Solid Edge part; units mm, degrees
sketch "Sketch1" plane through (0, 0, 0) normal (0, -1, 0) x (1, 0, 0)
  line L0 (-13.5, 0) -> (13.5, 0)
  line L1 (13.5, 0) -> (13.5, 90)
  line L2 (13.5, 90) -> (-13.5, 90)
  line L3 (-13.5, 90) -> (-13.5, 0)
  dimension "D1" = 13.5
  dimension "D2" = 13.5
extrude "Protrusion1" add sketch "Sketch1" against normal blind 17
sketch "Sketch2" plane through (0, 17, 40) normal (0, 1, 0) x (-1, 0, 0)
  line L0 (-10.5, -30) -> (10.5, -30)
  line L1 (10.5, -30) -> (10.5, 11)
  line L2 (10.5, 11) -> (-10.5, 11)
  line L3 (-10.5, 11) -> (-10.5, -30)
  dimension "D1" = 10.5
  dimension "D2" = 10.5
extrude "ExtrudedCutout_1" cut sketch "Sketch2" against normal blind 53.489
sketch "Sketch3" plane through (0, 17, 40) normal (0, 1, 0) x (-1, 0, 0)
  line L0 (-4.432, 40.7205) -> (-1.9698, 26.7205)
  arc A0 (-1.9698, 26.7205) -> (1.9698, 26.7205) centre (0, 27.067) ccw
  line L1 (4.432, 40.7205) -> (1.9698, 26.7205)
  arc A1 (-4.432, 40.7205) -> (4.432, 40.7205) centre (0, 41.5) cw
  dimension "D1" = 4.432
extrude "ExtrudedCutout_2" cut sketch "Sketch3" against normal blind 5
fillet "Round_1" radius 6 4 edges at (-13.5, 8.5, 0) (13.5, 8.5, 0) (13.5, 8.5, 90) (-13.5, 8.5, 90)
sketch "Sketch4" plane through (0, 12, 75.5335) normal (0, 1, 0) x (-0.1732, 0, -0.9849)
  circle A0 centre (-5.8763, 1.0335) radius 1
extrude "Cutout1" cut sketch "Sketch4" against normal through all
sketch "Sketch5" plane through (0, 0, 45) normal (0, -1, 0) x (0, 0, 1)
  circle A0 centre (36.5, 0) radius 4.5
extrude "ExtrudedCutout_4" cut sketch "Sketch5" against normal blind 8.5833
sketch "Sketch6" plane through (0, 0, 45) normal (0, -1, 0) x (0, 0, -1)
  line L0 (17.05, 13.5) -> (32.05, 13.5)
  line L1 (32.05, 13.5) -> (32.05, 10.5)
  line L2 (32.05, 10.5) -> (17.05, 10.5)
  line L3 (17.05, 10.5) -> (17.05, 13.5)
  line L4 (17.05, -10.5) -> (32.05, -10.5)
  line L5 (32.05, -10.5) -> (32.05, -13.5)
  line L6 (32.05, -13.5) -> (17.05, -13.5)
  line L7 (17.05, -13.5) -> (17.05, -10.5)
  dimension "D1" = 17.05
extrude "ExtrudedProtrusion_3" add sketch "Sketch6" along normal blind 12
sketch "Sketch7" plane through (-12, -12, 20.45) normal (0, -1, 0) x (0, 0, -1)
  line L0 (-7.5, -1.5) -> (7.5, -1.5)
  line L1 (7.5, -1.5) -> (7.5, 25.5)
  line L2 (7.5, 25.5) -> (-7.5, 25.5)
  line L3 (-7.5, 25.5) -> (-7.5, -1.5)
extrude "ExtrudedProtrusion_4" add sketch "Sketch7" along normal blind 3.4534
sketch "Sketch8" plane through (0, -15.4534, 20.45) normal (0, -1, 0) x (1, 0, 0)
  circle A0 centre (0, 0) radius 1.5
extrude "ExtrudedCutout_5" cut sketch "Sketch8" against normal blind 4.5945
fillet "Round_2" radius 6 3 edges at (-12, 0, 27.95) (12, 0, 27.95) (-12, 0, 12.95)
Input: part model. Units: mm. Frame: model coordinates. A direction names the side the tool comes from. Coordinates: 2 decimals unless noted, no trailing zeros. Loops run counter-clockwise (first coordinate to the right, second up) from the corner with the lowest first, then second, coordinate; pieces in that order, holes last. Notation, with made-up numbers: (75.25, -7) - (99.25, -7) arc R31 cw to (99.25, 28) - close; hole circle Ø10 at (66.5, 89). An arc over 180 degrees is marked (long way). Answer in a Markdown table with one row per item. Add a question column.
Item 1: Contact query for flat-ended pins moving along their axis: P1, Ø7.5, axis at x = -3, z = 22.5, coming from the +Y side; P2, Ø2.5, axis at x = 0, z = 81.5, coming from the -Y side; P3, Ø10, axis at x = 0, z = 82.5, coming from the -Y side. Output: stop coordinate, or through.
Item 2: Section query B-B on y = 3.5. Return the cut outline in (x, z).
Item 3: Section query C-C on x = 3.25. Return the cut outline in (y, z).
Item 4: Mould query, pull axis Z, two halves, no side actions, for faces 5 (the flat face through (0, -13, 27.95)), 6 (the flat face through (0, 8.583, 83)), 7 (the cylindrical face through (-11.696, 8.619, 1.711)). Classes: released by +Z, released by -Z, zero draft, split by the parting line, or undercut.
Item 5: Access query for faces 1 (the flat face through (0, 9, 51)), 2 (the flat face through (0, 0, 4)), 3 (the flat face through (-3.22, 14.54, 73.82)), 4 (the cylindrical face through (-11.789, 8.619, 88.196)). Directions: +Z, -Z, +X, -X, +Y, -Y. A direction counts if a zero-diameter tool reaches every point of the face in a straight line with its end or side. Return the directions, or none.
Item 6: Line query: line 1 along Z through (x, y) = (0, 2.5); line 2 along Z through (x, y) = (0, 15.15); line 3 along Z through (x, y) = (0, -13.75). Output: solid intervals per line, ascending. Write a range as [from, to].
Item 7: Section query A-A on z = 40.5. Return the cut outline in (x, y).
Item 8: Section query D-D on z = 20.45. Return the cut outline in (x, y), then the cut area to 3 significant figures.
Recorded:
| question | item | result |
|---|---|---|
| 1 | P1 | y = -12 |
| 1 | P2 | y = 8.58 |
| 1 | P3 | y = 0 |
| 2 | outline | (-13.5, 6) arc R6 ccw to (-7.5, 0) - (7.5, 0) arc R6 ccw to (13.5, 6) - (13.5, 84) arc R6 ccw to (7.5, 90) - (-7.5, 90) arc R6 ccw to (-13.5, 84) - close; hole (-10.5, 10) - (10.5, 10) - (10.5, 51) - (-10.5, 51) - close; hole circle Ø9 at (0, 81.5) |
| 3 | outline | (-15.45, 12.95) - (-12, 12.95) - (-12, 27.95) - (-15.45, 27.95) - close; (-0.83, 10) arc R6 cw to (0, 6.95) - (0, 0) - (17, 0) - (17, 10) - close; (0, 51) - (17, 51) - (17, 74) - (12, 74) - (12, 84.61) - (17, 84.61) - (17, 90) - (0, 90) - (0, 84.61) - (8.58, 84.61) - (8.58, 78.39) - (0, 78.39) - close |
| 4 | face 5 | released by +Z |
| 4 | face 6 | undercut |
| 4 | face 7 | released by -Z |
| 5 | face 1 | +Y, -Y |
| 5 | face 2 | -Z, +X, -X, -Y |
| 5 | face 3 | +Y |
| 5 | face 4 | +Z, -X, +Y, -Y |
| 6 | line 1 | [0, 10], [51, 77], [86, 90] |
| 6 | line 2 | [0, 10], [51, 65.07], [86, 90] |
| 6 | line 3 | [12.95, 18.95], [21.95, 27.95] |
| 7 | outline | (-13.5, 0) - (-10.5, 0) - (-10.5, 17) - (-13.5, 17) - close; (10.5, 0) - (13.5, 0) - (13.5, 17) - (10.5, 17) - close |
| 8 | outline | (-13.5, -15.45) - (-1.5, -15.45) - (-1.5, -12) - (-10.5, -12) - (-10.5, 17) - (-13.5, 17) - close; (1.5, -15.45) - (13.5, -15.45) - (13.5, 17) - (10.5, 17) - (10.5, -12) - (1.5, -12) - close |
| 8 | area | 257 mm^2 |
